Can you work these out from the model? Positions are in its coordinate system, mm. A direction names the side the tool comes from. Give positions to 0.01 mm unless a question says otherwise; leave off trailing zeros. Order: outer loops, then holes, each group sorted by start corner. A loop starts at its lowest first (then second) coordinate and runs counter-clockwise, first axis right, second up.
Item 1: Which directions (+Z, -Z, +X, -X, +Y, -Y) give clear straight access to the entire face, cutting with the end or side of a thin tool? Please do faces 1 (the flat face through (21, -11.049, 11)), 2 (the flat face through (21, 11.049, 11)), 3 (the cylindrical face through (15.33, -0.15, 13.83)).
Item 2: I'm going to push flat-ended pins straight in: pin 1 Ø4 at (x, z) = (5.5, -3.5) entering from +Y; pin 2 Ø6 at (y, z) = (-8, -27.5) entering from +X (3 decimals); pin 3 Ø11 at (x, z) = (27.5, 8) entering from -Y; pin 4 Ø6 at (y, z) = (3, -13) entering from -X. Where does each tip first touch, or does it pass through?
Item 3: I want a section at C-C, the plane x = 16.5. Write out the boundary of the cut face in (y, z).
Item 4: I want a section at D-D, the plane y = -4.5. Write out the boundary of the cut face in (x, z) (3 decimals), then the cut area to 3 significant figures.
Item 5: I want a section at A-A, the plane y = 2. Write out the boundary of the cut face in (x, z) (3 decimals).
Item 6: If we mould it in two halves opening along Y, with no side actions, what happens to faces 4 (the flat face through (2, 17.462, 1)), 5 (the flat face through (13.44, -0.15, 25.89)), 6 (the cylindrical face through (1.61, 0.15, -41.55)), 7 (the cylindrical face through (1.6, 0.1, -21.3))? For each: +Y half, -Y half, draft (parallel to the pull), parting line (faces both ways), or undercut.
Item 7: If I drill on line 1 along X through (y, z) = (-10, 42) (3 decimals); line 2 along Y through (x, z) = (15.5, 16); line 3 along X through (y, z) = (10, 10.5), over which ranges is the centre line in solid material (lowest first)?
Item 8: I want a section at B-B, the plane z = 45.5. Write out the boundary of the cut face in (x, y) (1 decimal), then the cut area to 3 significant figures.
```python
from build123d import *

# Parameters (mm, degrees)
SKETCH1_W               = 107.95
SKETCH1_H               = 34.925
BOSS_EXTRUDE1_DEPTH     = 3.175
BOSS_EXTRUDE2_REACH     = 92.429
SKETCH4_W               = 22.098
SKETCH4_H               = 22.098
CUT_EXTRUDE1_REACH      = 69.122
SKETCH5_R               = 3.3782
F_1_4_20_TAPPED_HOLE1_D = 5.1054


with BuildPart() as part:
    # Sketch1 → Boss-Extrude1 (new body)
    with BuildSketch(Plane(origin=(0, 0, 0), x_dir=(0, 0, -1), z_dir=(1, 0, 0))):
        Rectangle(SKETCH1_W, SKETCH1_H)
    extrude(amount=BOSS_EXTRUDE1_DEPTH)

    # Boss-Extrude2: up to this plane
    boss_extrude2_end = Plane(origin=(3.175, 0, 0), z_dir=(1, 0, 0))
    # Sketch4 → Boss-Extrude2 (add, up to the surface)
    with BuildSketch(Plane(origin=(29.650800378, 0, 29.650800378), x_dir=(0.707106781186546, 0, -0.707106781186549), z_dir=(0.707106781186549, 0, 0.707106781186546)), mode=Mode.PRIVATE) as boss_extrude2_sk1:
        with Locations((2.24506403, 0)):
            Rectangle(SKETCH4_W, SKETCH4_H)
    boss_extrude2_tool1 = split(extrude(boss_extrude2_sk1.sketch, amount=-BOSS_EXTRUDE2_REACH, mode=Mode.PRIVATE), bisect_by=boss_extrude2_end, keep=Keep.BOTH, mode=Mode.PRIVATE)
    add(boss_extrude2_tool1.solids().sort_by_distance((31.2383, 0, 28.0633))[0])

    # Sketch5 → Cut-Extrude1 (cut, up to next)
    with BuildSketch(Plane(origin=(3.175, 0, 0), x_dir=(0, 0, -1), z_dir=(1, 0, 0)), mode=Mode.PRIVATE) as cut_extrude1_sk1:
        with Locations((-44.925561602, 0)):
            Circle(SKETCH5_R)
    cut_extrude1_tool1 = extrude(cut_extrude1_sk1.sketch, amount=-CUT_EXTRUDE1_REACH, mode=Mode.PRIVATE) & part.part
    # Sketch5 → Cut-Extrude1 (cut, up to next)
    with BuildSketch(Plane(origin=(3.175, 0, 0), x_dir=(0, 0, -1), z_dir=(1, 0, 0)), mode=Mode.PRIVATE) as cut_extrude1_sk2:
        with Locations((24.675084049, 0)):
            Circle(SKETCH5_R)
    cut_extrude1_tool2 = extrude(cut_extrude1_sk2.sketch, amount=-CUT_EXTRUDE1_REACH, mode=Mode.PRIVATE) & part.part
    # Sketch5 → Cut-Extrude1 (cut, up to next)
    with BuildSketch(Plane(origin=(3.175, 0, 0), x_dir=(0, 0, -1), z_dir=(1, 0, 0)), mode=Mode.PRIVATE) as cut_extrude1_sk3:
        with Locations((44.925561602, 0)):
            Circle(SKETCH5_R)
    cut_extrude1_tool3 = extrude(cut_extrude1_sk3.sketch, amount=-CUT_EXTRUDE1_REACH, mode=Mode.PRIVATE) & part.part
    add(cut_extrude1_tool1.solids().sort_by_distance((3.175, 0, 44.925562))[0], mode=Mode.SUBTRACT)
    add(cut_extrude1_tool2.solids().sort_by_distance((3.175, 0, -24.675084))[0], mode=Mode.SUBTRACT)
    add(cut_extrude1_tool3.solids().sort_by_distance((3.175, 0, -44.925562))[0], mode=Mode.SUBTRACT)

    # 1/4-20 Tapped Hole1 (through all)
    with Locations(Plane(origin=(0, 11.049, 0), x_dir=(1, 0, 0), z_dir=(0, 1, 0))):
        with Locations((17.767916197, -14.592916197), (26.748172318, -23.573172318)):
            Hole(F_1_4_20_TAPPED_HOLE1_D / 2)


solid = part.part
```
Results list:
1. face 1: +Z, -Z, +X, -Y
1. face 2: +Z, -Z, +X, +Y
1. face 3: +Y, -Y
2. pin 1: stops at y = 11.05
2. pin 2: stops at x = 3.175
2. pin 3: stops at y = -11.05
2. pin 4: stops at x = 0
3. outline: (-11.05, -2.3) - (11.05, -2.3) - (11.05, 12.38) - (-11.05, 12.38) - close; (-11.05, 16.81) - (11.05, 16.81) - (11.05, 28.95) - (-11.05, 28.95) - close
4. outline: (0, -53.975) - (3.175, -53.975) - (3.175, -15.626) - (39.051, 20.25) - (23.425, 35.876) - (3.175, 15.626) - (3.175, 53.975) - (0, 53.975) - close; hole circle Ø5.105 at (17.768, 14.593); hole circle Ø5.105 at (26.748, 23.573)
4. area: 1,180 mm2
5. outline: (0, -53.975) - (3.175, -53.975) - (3.175, -47.648) - (0, -47.648) - close; (0, -42.203) - (3.175, -42.203) - (3.175, -27.398) - (0, -27.398) - close; (0, -21.953) - (3.175, -21.953) - (3.175, -15.626) - (39.051, 20.25) - (23.425, 35.876) - (3.175, 15.626) - (3.175, 42.203) - (0, 42.203) - close; (0, 47.648) - (3.175, 47.648) - (3.175, 53.975) - (0, 53.975) - close; hole circle Ø5.105 at (17.768, 14.593); hole circle Ø5.105 at (26.748, 23.573)
6. face 4: +Y half
6. face 5: draft
6. face 6: undercut
6. face 7: undercut
7. line 1: x = 0 to 3.175
7. line 2: y = -11.05 to 11.05
7. line 3: x = 0 to 29.3
8. outline: (0, -17.5) - (3.2, -17.5) - (3.2, -3.3) - (0, -3.3) - close; (0, 3.3) - (3.2, 3.3) - (3.2, 17.5) - (0, 17.5) - close
8. area: 89.7 mm2
